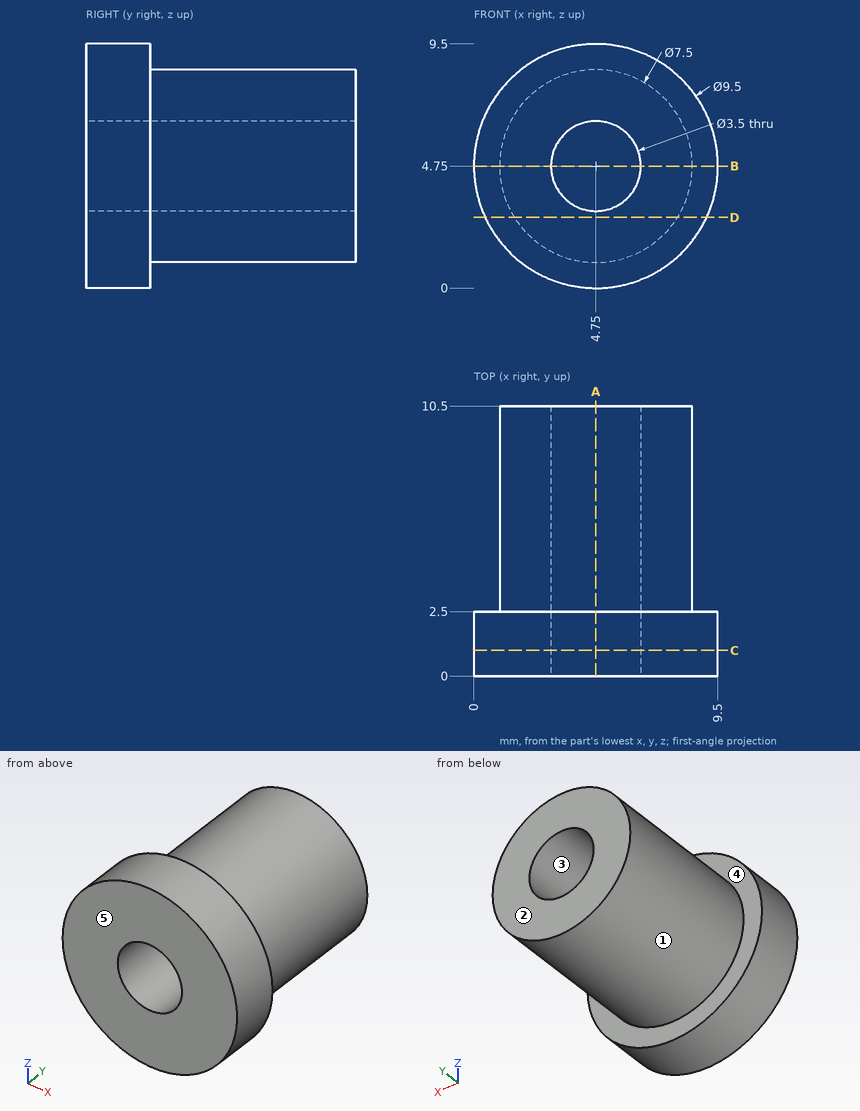
Check sheet for the drawn part. Datum: minimum x, y, z corner. Units: mm. A direction names the side the tool comes from. Give positions to 0.01 mm unless a question says otherwise; leave off trailing zeros. Order: outer loops, then holes, each group sorted by start corner. A loop starts at its lowest first (then second) coordinate and runs counter-clockwise, first axis right, second up. Notation, with made-up numbers: (59.5, 60) -> (102.5, 60) arc R29 ccw to (102.5, 91) -> close; hole circle Ø7 at (-3, 3). An arc over 180 degrees is marked (long way). One line per item, written item: value.
(1) Gauge pin test, flat ends, axial feed: pin 1 (4 mm diameter, centred on y = 7.5, z = 2.5, fed in from +X); pin 2 (4.5 mm diameter, centred on x = 4.75, z = 4.75, fed in from +Y); pin 3 (3 mm diameter, centred on y = 8.5, z = 2.5, fed in from -X); pin 4 (1 mm diameter, centred on y = 4, z = 4, fed in from -X). Record the tip position at first contact, or that the pin passes through.
Final values:
pin 1: x = 8.49
pin 2: y = 10.5
pin 3: x = 1.08
pin 4: x = 1.01
(2) Draft check along X on the marked faces 1, 2 and 3. Enter one of: pulls with the +X half, pulls with the -X half, needs draft (parallel to the pull), parting line crosses it, or undercut.
Final values:
face 1: parting line crosses it
face 2: needs draft
face 3: undercut
(3) Sectioned sample at B-B on z = 4.75. Record the cut outline in (x, y), then the cut area to 3 significant figures.
Final values:
outline: (0, 0) -> (3, 0) -> (3, 10.5) -> (1, 10.5) -> (1, 2.5) -> (0, 2.5) -> close; (6.5, 0) -> (9.5, 0) -> (9.5, 2.5) -> (8.5, 2.5) -> (8.5, 10.5) -> (6.5, 10.5) -> close
area: 47.0 mm^2
(4) Tool access check on the marked faces 4 and 5. Record the directions out of +Z, -Z, +X, -X, +Y, -Y that give a thin tool (end or side, any length) a straight path to the whole face; none if there is none.
Final values:
face 4: +Y
face 5: +Z, -Z, +X, -X, -Y
(5) Scan lines: line 1 along Z through (x, y) = (4.75, 4.25); line 2 along Y through (x, z) = (1, 5.25). Record each from-to range of solid material in increasing order. Write a range as [from, to].
Final values:
line 1: [1, 3], [6.5, 8.5]
line 2: [0, 2.5]
(6) Sectioned sample at C-C on y = 1. Record the cut outline in (x, z).
Final values:
outline: circle Ø9.5 at (4.75, 4.75); hole circle Ø3.5 at (4.75, 4.75)
(7) Sectioned sample at A-A on x = 4.75. Record the cut outline in (y, z), then the cut area to 3 significant figures.
Final values:
outline: (0, 0) -> (2.5, 0) -> (2.5, 1) -> (10.5, 1) -> (10.5, 3) -> (0, 3) -> close; (0, 6.5) -> (10.5, 6.5) -> (10.5, 8.5) -> (2.5, 8.5) -> (2.5, 9.5) -> (0, 9.5) -> close
area: 47.0 mm^2
(8) Sectioned sample at D-D on z = 2.75. Record the cut outline in (x, y), then the cut area to 3 significant figures.
Final values:
outline: (0.44, 0) -> (9.06, 0) -> (9.06, 2.5) -> (7.92, 2.5) -> (7.92, 10.5) -> (1.58, 10.5) -> (1.58, 2.5) -> (0.44, 2.5) -> close
area: 72.3 mm^2
